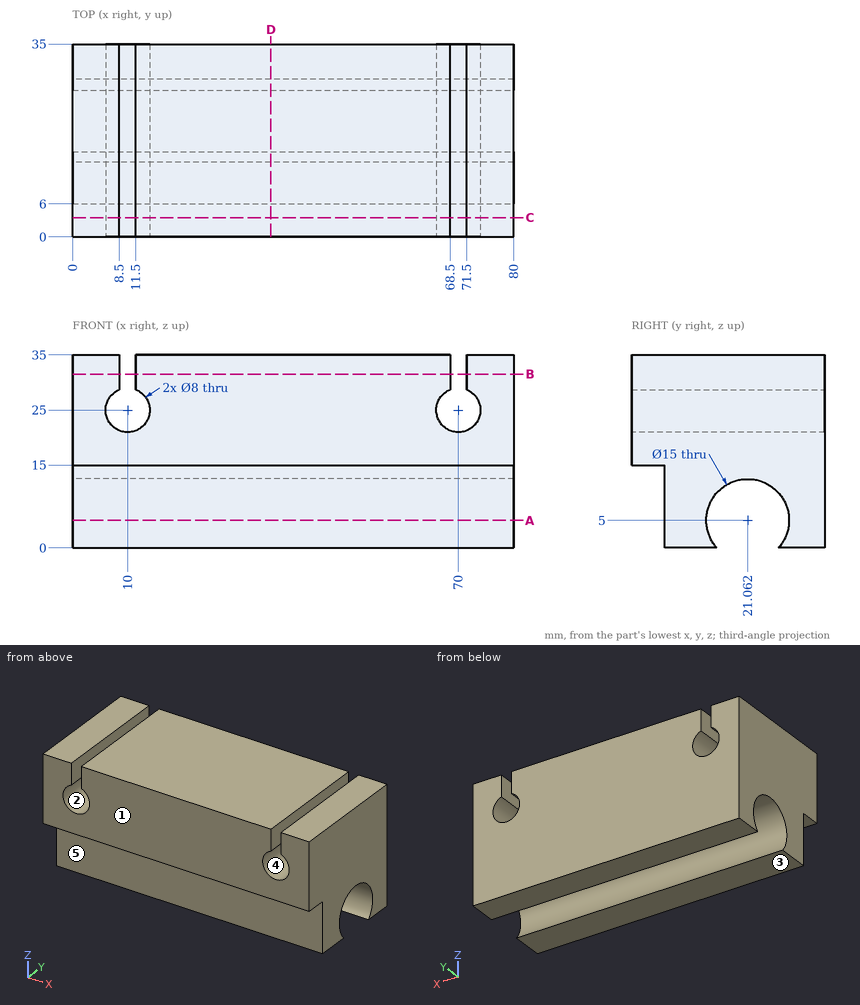
Geometry: see drawing. Coordinates: mm, zero at the bounding-box minimum. A direction names the side the tool comes from. Coordinates: 2 decimals unless noted, no trailing zeros. Loops run counter-clockwise (first coordinate to the right, second up) from the corner with the lowest first, then second, coordinate; pieces in that order, holes last.
Q1. Cut plane C-C (y = 3.5). Output: boundary loops of the cut face in (x, z).
Q2. Cut plane D-D (x = 36). Output: boundary loops of the cut face in (y, z), then the cut area to 3 significant figures.
Q3. Cut plane A-A (z = 5). Output: boundary loops of the cut face in (x, y).
Q4. Draft query along Z for the marked faces 1, 2 and 3. Return one class per face: +Z half, -Z half, draft (parallel to the pull), parting line (faces both ways), or undercut.
Q5. Cut plane B-B (z = 31.5). Output: boundary loops of the cut face in (x, y), then the cut area to 3 significant figures.
Q6. Contact query for flat-ended pins moving along their axis: pin 1 (9 mm diameter, centred on x = 70, z = 25, fed in from +Y); pin 2 (13.5 mm diameter, centred on y = 21.062, z = 5, fed in from +X); pin 3 (5 mm diameter, centred on x = 57, y = 3, fed in from -Z). Output: stop coordinate, or through.
Q7. Set-up query: the marked faces 4 and 5. Return all of +Z, -Z, +X, -X, +Y, -Y with unobstructed straight access to the full face (end or side cutting, diameter ignored); none if empty.
Q8. Material intervals for line 1 (X direction, y = 27, z = 25); line 2 (Y direction, x = 50, z = 5); line 3 (X direction, y = 10, z = 22), sorted ascending.
Working result:
1. outline: (0, 15) - (80, 15) - (80, 35) - (71.5, 35) - (71.5, 28.71) arc R4 cw (long way) to (68.5, 28.71) - (68.5, 35) - (11.5, 35) - (11.5, 28.71) arc R4 cw (long way) to (8.5, 28.71) - (8.5, 35) - (0, 35) - close
2. outline: (0, 15) - (6, 15) - (6, 0) - (15.47, 0) arc R7.5 cw (long way) to (26.65, 0) - (35, 0) - (35, 35) - (0, 35) - close
2. area: 978 mm2
3. outline: (0, 6) - (80, 6) - (80, 13.56) - (0, 13.56) - close; (0, 28.56) - (80, 28.56) - (80, 35) - (0, 35) - close
4. face 1: draft
4. face 2: undercut
4. face 3: -Z half
5. outline: (0, 0) - (8.5, 0) - (8.5, 35) - (0, 35) - close; (11.5, 0) - (68.5, 0) - (68.5, 35) - (11.5, 35) - close; (71.5, 0) - (80, 0) - (80, 35) - (71.5, 35) - close
5. area: 2,590 mm2
6. pin 1: stops at y = 35
6. pin 2: passes through
6. pin 3: stops at z = 15
7. face 4: +Y, -Y
7. face 5: -Z, +X, -X, -Y
8. line 1: x = 0 to 6, 14 to 66, 74 to 80
8. line 2: y = 6 to 13.56, 28.56 to 35
8. line 3: x = 0 to 7.35, 12.65 to 67.35, 72.65 to 80
